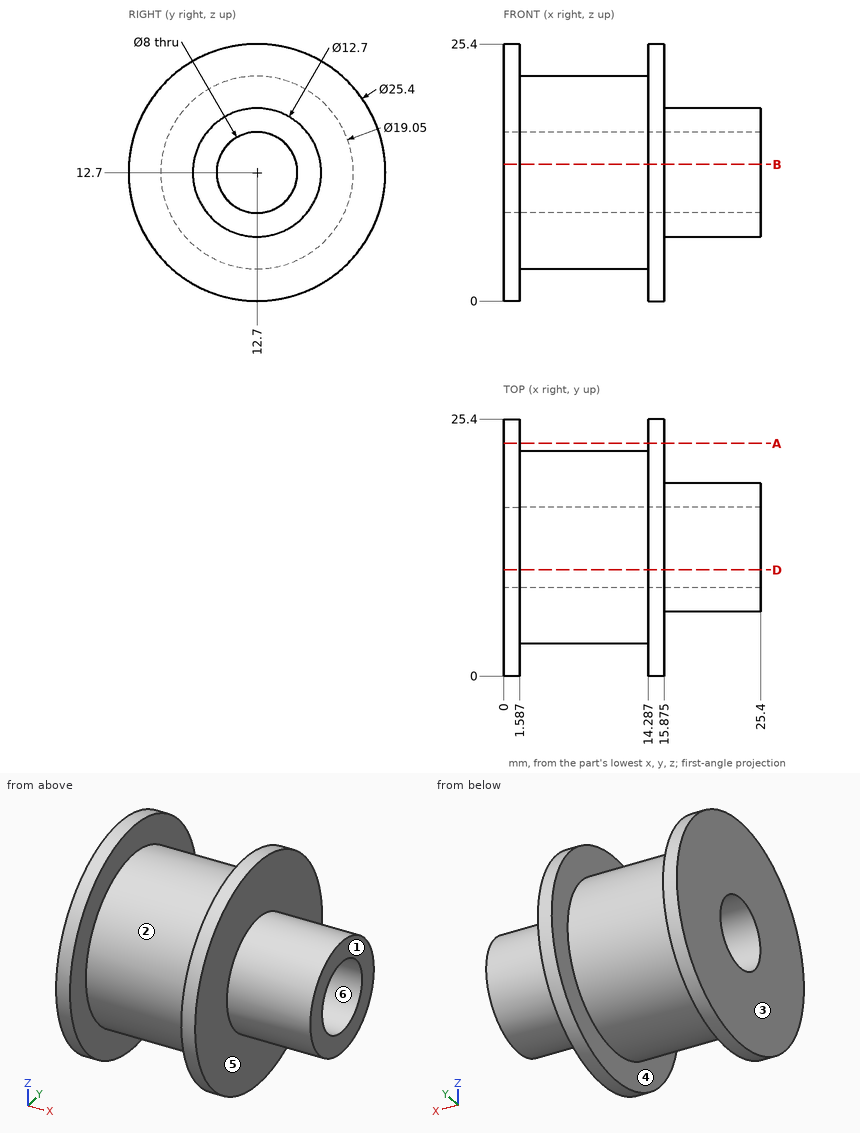
Input: dimensioned drawing with shaded views. Units: mm. Origin: part minimum x, y, z. A direction names the side the tool comes from. Give positions to 0.01 mm unless a question says otherwise; leave off trailing zeros. Write each loop counter-clockwise with the first axis right and the second up, starting at its lowest first coordinate (ties: lowest second). Pieces come first, ordered by that corner, then holes. Notation, with made-up numbers: M 54.25,8.25 L 75.25,8.25 A28 ccw 75.25,47.25 Z; hole C -15,-28 d6. An arc over 180 degrees is marked long. Return JSON: item names as keys, results as strings. Group by question number.
1) Cut plane D-D, the plane y = 10.5. Output: boundary loops of the cut face in (x, z) (1 decimal).
2) Cut plane B-B, the plane z = 13.5. Output: boundary loops of the cut face in (x, y) (1 decimal).
3) Pin query (flat end, axial travel): P1, Ø2, axis at x = 11, z = 17.5, coming from the +Y side (1 decimal); P2, Ø2, axis at x = 4, z = 3, coming from the +Y side (1 decimal); P3, Ø10, axis at x = 16, y = 19, coming from the +Z side; P4, Ø6.5, axis at y = 12.7, z = 12.7, coming from the +X side. Return the tip coordinate at first contact, or that it passes through.
4) Cut plane A-A, the plane y = 23. Output: boundary loops of the cut face in (x, z) (1 decimal).
5) Material intervals for line 1 along Y through (x, z) = (10.25, 12.5) (1 decimal); line 2 along X through (y, z) = (12, 24.25) (1 decimal); line 3 along Y through (x, z) = (19.5, 12.7), sorted ascending. Write a range as [from, to].
6) Set-up query: the marked faces 4, 5 and 6. Return all of +Z, -Z, +X, -X, +Y, -Y with unobstructed straight access to the full face (end or side cutting, diameter ignored); none if empty.
7) Pull-direction query (X, two-part tool) for the marked faces 1, 2 and 3; classes: pulls with the +X half, pulls with the -X half, needs draft (parallel to the pull), parting line crosses it, or undercut.
Recorded:
{
 "1": {"outline": "M 0,0.2 L 1.6,0.2 L 1.6,3.4 L 14.3,3.4 L 14.3,0.2 L 15.9,0.2 L 15.9,6.7 L 25.4,6.7 L 25.4,9.4 L 0,9.4 Z; M 0,16 L 25.4,16 L 25.4,18.7 L 15.9,18.7 L 15.9,25.2 L 14.3,25.2 L 14.3,22 L 1.6,22 L 1.6,25.2 L 0,25.2 Z"},
 "2": {"outline": "M 0,0 L 1.6,0 L 1.6,3.2 L 14.3,3.2 L 14.3,0 L 15.9,0 L 15.9,6.4 L 25.4,6.4 L 25.4,8.8 L 0,8.8 Z; M 0,16.6 L 25.4,16.6 L 25.4,19 L 15.9,19 L 15.9,25.4 L 14.3,25.4 L 14.3,22.2 L 1.6,22.2 L 1.6,25.4 L 0,25.4 Z"},
 "3": {"P1": "stops at y = 21.4", "P2": "stops at y = 16.6", "P3": "stops at z = 25.33", "P4": "passes through"},
 "4": {"outline": "M 0,5.3 L 1.6,5.3 L 1.6,20.1 L 0,20.1 Z; M 14.3,5.3 L 15.9,5.3 L 15.9,20.1 L 14.3,20.1 Z"},
 "5": {"line 1": "y = [3.2, 8.7], [16.7, 22.2]", "line 2": "x = [0, 1.6], [14.3, 15.9]", "line 3": "y = [6.35, 8.7], [16.7, 19.05]"},
 "6": {"face 4": "none", "face 5": "+X", "face 6": "+X, -X"},
 "7": {"face 1": "pulls with the +X half", "face 2": "undercut", "face 3": "pulls with the -X half"}
}
